Autodesk Inventor part; units mm, degrees
ref_plane "YZ Plane" through (0, 0, 0) normal (1, 0, 0) x (0, 1, 0)
ref_plane "XZ Plane" through (0, 0, 0) normal (0, 1, 0) x (-1, 0, 0)
ref_plane "XY Plane" through (0, 0, 0) normal (0, 0, 1) x (1, 0, 0)
ref_plane "Płaszczyzna konstrukcyjna1" through (0, 0, 0) normal (0, 0, 1) x (1, 0, 0)
sketch "Szkic1" plane through (0, 0, 0) normal (0, 0, 1) x (1, 0, 0)
  circle A0 centre (-437.5, -300) radius 4
  circle A1 centre (-437.5, 300) radius 4
  circle A2 centre (-300, 437.5) radius 4
  circle A3 centre (300, 437.5) radius 4
  circle A4 centre (437.5, 300) radius 4
  circle A5 centre (437.5, -300) radius 4
  circle A6 centre (-437.5, 0) radius 4
  circle A7 centre (0, 437.5) radius 4
  circle A8 centre (437.5, 0) radius 4
  circle A9 centre (300, -437.5) radius 4
  circle A10 centre (-300, -437.5) radius 4
  circle A11 centre (0, -437.5) radius 4
  line L0 (398.5, -398.5) -> (398.5, 398.5)
  line L1 (-398.5, -398.5) -> (398.5, -398.5)
  line L2 (-398.5, 398.5) -> (-398.5, -398.5)
  line L3 (398.5, 398.5) -> (-398.5, 398.5)
  line L4 (-457.5, -457.5) -> (-457.5, 457.5)
  line L5 (457.5, -457.5) -> (-457.5, -457.5)
  line L6 (457.5, 457.5) -> (457.5, -457.5)
  line L7 (-457.5, 457.5) -> (457.5, 457.5)
  line L8 (437.5, -437.5) -> (-437.5, -437.5)
  line L9 (-437.5, -437.5) -> (-437.5, 437.5)
  line L10 (-437.5, 437.5) -> (437.5, 437.5)
  line L11 (437.5, 437.5) -> (437.5, -437.5)
  line L12 (437.5, -437.5) -> (-437.5, 437.5) construction
  line L13 (-437.5, -437.5) -> (437.5, 437.5) construction
  circle A12 centre (-437.5, 300) radius 17.5
  circle A13 centre (-437.5, 0) radius 17.5
  circle A14 centre (-437.5, -300) radius 17.5
  circle A15 centre (-422.5, 422.5) radius 3
  circle A16 centre (-422.5, 362.5) radius 3
  circle A17 centre (-422.5, 250) radius 3
  circle A18 centre (-422.5, 150) radius 3
  circle A19 centre (-422.5, 50) radius 3
  line L14 (-437.5, 0) -> (437.5, 0) construction
  circle A20 centre (-422.5, -362.5) radius 3
  circle A21 centre (-422.5, -250) radius 3
  circle A22 centre (-422.5, -150) radius 3
  circle A23 centre (-422.5, -50) radius 3
  circle A24 centre (0, -437.5) radius 17.5
  circle A25 centre (-50, -422.5) radius 3
  circle A26 centre (-250, -422.5) radius 3
  line L15 (437.5, -437.5) -> (-437.5, -437.5)
  line L16 (0, -437.5) -> (0, 437.5) construction
  line L17 (437.5, 437.5) -> (-437.5, -437.5) construction
  circle A27 centre (50, -422.5) radius 3
  circle A28 centre (-150, -422.5) radius 3
  circle A29 centre (-422.5, -422.5) radius 3
  circle A30 centre (250, -422.5) radius 3
  circle A31 centre (362.5, -422.5) radius 3
  circle A32 centre (-362.5, -422.5) radius 3
  circle A33 centre (-300, -437.5) radius 17.5
  circle A34 centre (300, -437.5) radius 17.5
  circle A35 centre (150, -422.5) radius 3
  circle A36 centre (437.5, 0) radius 17.5
  circle A37 centre (422.5, -50) radius 3
  circle A38 centre (422.5, -250) radius 3
  line L18 (437.5, 437.5) -> (437.5, -437.5)
  line L19 (437.5, 0) -> (-437.5, 0) construction
  line L20 (-437.5, 437.5) -> (437.5, -437.5) construction
  circle A39 centre (422.5, 50) radius 3
  circle A40 centre (422.5, -150) radius 3
  circle A41 centre (422.5, -422.5) radius 3
  circle A42 centre (422.5, 250) radius 3
  circle A43 centre (422.5, 362.5) radius 3
  circle A44 centre (422.5, -362.5) radius 3
  circle A45 centre (437.5, -300) radius 17.5
  circle A46 centre (437.5, 300) radius 17.5
  circle A47 centre (422.5, 150) radius 3
  circle A48 centre (0, 437.5) radius 17.5
  circle A49 centre (50, 422.5) radius 3
  circle A50 centre (250, 422.5) radius 3
  line L21 (-437.5, 437.5) -> (437.5, 437.5)
  line L22 (0, 437.5) -> (0, -437.5) construction
  line L23 (-437.5, -437.5) -> (437.5, 437.5) construction
  circle A51 centre (-50, 422.5) radius 3
  circle A52 centre (150, 422.5) radius 3
  circle A53 centre (422.5, 422.5) radius 3
  circle A54 centre (-250, 422.5) radius 3
  circle A55 centre (-362.5, 422.5) radius 3
  circle A56 centre (362.5, 422.5) radius 3
  circle A57 centre (300, 437.5) radius 17.5
  circle A58 centre (-300, 437.5) radius 17.5
  circle A59 centre (-150, 422.5) radius 3
  circle A60 centre (-362.5, 422.5) radius 3
  circle A61 centre (50, 422.5) radius 3
  circle A62 centre (422.5, 422.5) radius 3
  circle A63 centre (422.5, 50) radius 3
  circle A64 centre (422.5, -362.5) radius 3
  circle A65 centre (150, -422.5) radius 3
  circle A66 centre (-250, -422.5) radius 3
  circle A67 centre (-422.5, -250) radius 3
  circle A68 centre (-422.5, 150) radius 3
  circle A69 centre (-422.5, 50) radius 3
  circle A70 centre (-422.5, -362.5) radius 3
  circle A71 centre (-150, -422.5) radius 3
  circle A72 centre (250, -422.5) radius 3
  circle A73 centre (422.5, -250) radius 3
  circle A74 centre (422.5, 150) radius 3
  circle A75 centre (362.5, 422.5) radius 3
  circle A76 centre (-50, 422.5) radius 3
  circle A77 centre (-422.5, 422.5) radius 3
  circle A78 centre (-250, 422.5) radius 3
  circle A79 centre (150, 422.5) radius 3
  circle A80 centre (422.5, 362.5) radius 3
  circle A81 centre (422.5, -50) radius 3
  circle A82 centre (422.5, -422.5) radius 3
  circle A83 centre (50, -422.5) radius 3
  circle A84 centre (-362.5, -422.5) radius 3
  circle A85 centre (-422.5, -150) radius 3
  circle A86 centre (-422.5, 250) radius 3
  circle A87 centre (-422.5, -50) radius 3
  circle A88 centre (-422.5, -422.5) radius 3
  circle A89 centre (-50, -422.5) radius 3
  circle A90 centre (362.5, -422.5) radius 3
  circle A91 centre (422.5, -150) radius 3
  circle A92 centre (422.5, 250) radius 3
  circle A93 centre (250, 422.5) radius 3
  circle A94 centre (-150, 422.5) radius 3
  circle A95 centre (-422.5, 362.5) radius 3
  point P0 (0, 0)
  point P1 (0, 0)
  point P2 (0, 0)
  point P3 (0, 0)
  point P4 (-282.5, 437.5)
  point P5 (-317.5, 437.5)
  point P6 (-437.5, 317.5)
  point P7 (-437.5, 282.5)
  point P8 (-437.5, 17.5)
  point P9 (-437.5, -17.5)
  point P10 (-437.5, -282.5)
  point P11 (-437.5, -317.5)
  point P12 (-317.5, -437.5)
  point P13 (-282.5, -437.5)
  point P14 (-17.5, -437.5)
  point P15 (17.5, -437.5)
  point P16 (282.5, -437.5)
  point P17 (317.5, -437.5)
  point P18 (437.5, -317.5)
  point P19 (437.5, -282.5)
  point P20 (437.5, -17.5)
  point P21 (437.5, 17.5)
  point P22 (437.5, 282.5)
  point P23 (437.5, 317.5)
  point P24 (317.5, 437.5)
  point P25 (282.5, 437.5)
  point P26 (17.5, 437.5)
  point P27 (-17.5, 437.5)
  dimension "d0" = 875
  dimension "d1" = 35
  dimension "d4" = 300
  dimension "d9" = 6
  dimension "d10" = 15
  dimension "d11" = 6
  dimension "d12" = 15
  dimension "d13" = 60
  dimension "d14" = 6
  dimension "d15" = 6
  dimension "d16" = 6
  dimension "d17" = 100
  dimension "d18" = 100
  dimension "d19" = 15
  dimension "d20" = 15
  dimension "d21" = 15
  dimension "d22" = 50
  dimension "d25" = 360
extrude "Wyciągnięcie proste1" add sketch "Szkic1" along normal blind 3 contours L9 A13 A12 L10 A58 A48 A57 L11 A46 A36 A45 L8 A34 A24 A33 A14 | L1 L2 L3 L0
sketch "Szkic2" plane through (0, 0, 3) normal (0, 0, 1) x (1, 0, 0)
  circle A0 centre (-300, -300) radius 75
  point P0 (0, 0)
  dimension "d29" = 150
  dimension "d30" = 300
  dimension "d31" = 300
extrude "Wyciągnięcie proste2" cut sketch "Szkic2" against normal blind 3
properties part number "glas" material "Tworzywo, przezroczyste"
Geometry: final body of the model. Coordinates: model frame, mm. Round coordinates to 2 decimals unless told otherwise and drop trailing zeros. Order: outer loops, then holes, each group sorted by start corner. A loop starts at its lowest first (then second) coordinate and runs counter-clockwise, first axis right, second up. Notation, with made-up numbers: (-7, 81.5) - (23, 81.5) arc R33 cw to (23, 116.5) - close; hole circle Ø4 at (13, 37). An arc over 180 degrees is marked (long way). Use CSV: the item, a comma, the result in double quotes. Start each with the question number.
Q1. Mould query, pull axis X, two halves, no side actions, for faces 1 (the face through (-228.463, -277.472, 1.521)), 2 (the face through (-6, 6, 3)). Classes: +X half, -X half, draft (parallel to the pull), parting line (faces both ways), or undercut.
Q2. Material intervals for line 1 along X through (y, z) = (150, 1.9); line 2 along X through (y, z) = (-354.5, 2.1), sorted ascending. Write a range as from..to.
Q3. Section query A-A (z = 0.45). State how many separate pieces and enclosed holes the cut face has, and give its area (3 significant figures).
Q4. Section query B-B (x = 300). Return loops of the section in (y, z).
Q5. First-contact query: pin 1 (9.5 mm diameter, centred on x = 422.5, y = -362.5, fed in from +Z). Flat tip, straight axial feed; report the tip coordinate or a pass-through.
Result set:
1,face 1,"undercut"
1,face 2,"draft"
2,line 1,"x = -437.5..-425.5, -419.5..419.5, 425.5..437.5"
2,line 2,"x = -437.5..-351.52, -248.48..437.5"
3,separate pieces,"1"
3,enclosed holes,"37"
3,area,"741,000 mm2"
4,outline,"(-420, 0) - (420, 0) - (420, 3) - (-420, 3) - close"
5,pin 1,"stops at z = 3"
